Can you work these out from the model? Positions are in its coordinate system, mm. Round coordinates to 2 decimals unless told otherwise and drop trailing zeros. Loops run counter-clockwise (first coordinate to the right, second up) from the corner with the lowest first, then second, coordinate; pieces in that order, holes last. Notation, with made-up numbers: (16.5, -39.5) -> (75.5, -39.5) arc R28 ccw to (75.5, -15.5) -> close; hole circle Ø3 at (32.25, 39). An arc over 180 degrees is marked (long way). Write each question's results on one line, items separated by ' | '.
Autodesk Inventor part; units mm, degrees
ref_plane "YZ Plane" through (0, 0, 0) normal (1, 0, 0) x (0, 1, 0)
ref_plane "XZ Plane" through (0, 0, 0) normal (0, 1, 0) x (-1, 0, 0)
ref_plane "XY Plane" through (0, 0, 0) normal (0, 0, 1) x (1, 0, 0)
sketch "草圖1" plane through (0, 0, 0) normal (1, 0, 0) x (0, 1, 0)
  line L0 (-25, 50) -> (25, 50)
  line L1 (25, 50) -> (25, -50)
  line L2 (25, -50) -> (-25, -50)
  line L3 (-25, -50) -> (-25, 50)
  line L4 (-25, 50) -> (25, -50) construction
  line L5 (25, 50) -> (-25, -50) construction
  point P0 (0, 0)
  dimension "d0" = 50
  dimension "d1" = 100
extrude "擠出1" add sketch "草圖1" along normal blind 10
fillet "圓角1" radius 1 4 edges at (5, 25, 50) (5, -25, 50) (5, 25, -50) (5, -25, -50)
chamfer "倒角1" distance 1 angle 45 8 edges at (10, -25, 0) (10, -24.7071, -49.7071) (10, 0, -50) (10, 24.7071, -49.7071) (10, 25, 0) (10, 24.7071, 49.7071) (10, 0, 50) (10, -24.7071, 49.7071)
sketch "草圖2" plane through (10, 0, 0) normal (1, 0, 0) x (0, 0, -1)
  line L0 (-50, 24) -> (-50, -24)
  line L1 (49, 25) -> (-49, 25)
  line L2 (-30, 24) -> (-30, -24)
  line L3 (50, -24) -> (50, 24)
  line L4 (30, -24) -> (30, 24)
  line L5 (30, -12.5) -> (-30, -12.5)
  line L6 (-30, -12.5) -> (-30, 12.5)
  line L7 (-30, 12.5) -> (30, 12.5)
  line L8 (30, 12.5) -> (30, -12.5)
  line L9 (30, -12.5) -> (-30, 12.5) construction
  line L10 (-30, -12.5) -> (30, 12.5) construction
  point P0 (0, 0)
  dimension "d8" = 20
  dimension "d9" = 20
  dimension "d10" = 25
hole "孔1" at (10, 12.5, 30) at (10, -12.5, 30) at (10, 12.5, -30) at (10, -12.5, -30) direction (-1, 0, 0) diameter 10 end through all
thread "螺紋1"
thread "螺紋2"
chamfer "倒角2" distance 0.5 angle 45 8 edges at (10, -12.5, -25) (10, 12.5, -25) (10, -12.5, 35) (10, 12.5, 35) (0, -12.5, -25) (0, 12.5, -25) (0, -12.5, 35) (0, 12.5, 35)
properties part number "exercise3-3"
1. Please list where these lines run through material, in increasing order: line 1 (Y direction, x = 2.75, z = -30); line 2 (Z direction, x = 5.5, y = -12.5); line 3 (Z direction, x = 2.5, y = 10). Write a range as from..to.
Final values:
line 1: -25..-17.5, -7.5..7.5, 17.5..25 | line 2: -50..-35, -25..25, 35..50 | line 3: -50..-34.33, -25.67..25.67, 34.33..50
2. We'd pull the mould along Y, two halves only. Please class faces 1 (the face through (4, -25, -1)), 2 (the face through (4.937, -12.72, -25.005)), 3 (the face through (10, 0, 1)): pulls with the +Y half, pulls with the -Y half, needs draft (parallel to the pull), parting line crosses it, or undercut.
Final values:
face 1: pulls with the -Y half | face 2: undercut | face 3: needs draft
3. If we section it at A-A (z = -30): List the corners of the cut face in (x, y) for me, then the cut area to 3 significant figures.
Final values:
outline: (0, -25) -> (9, -25) -> (10, -24) -> (10, -18) -> (9.5, -17.5) -> (0.5, -17.5) -> (0, -18) -> close; (0, -7) -> (0.5, -7.5) -> (9.5, -7.5) -> (10, -7) -> (10, 7) -> (9.5, 7.5) -> (0.5, 7.5) -> (0, 7) -> close; (0, 18) -> (0.5, 17.5) -> (9.5, 17.5) -> (10, 18) -> (10, 24) -> (9, 25) -> (0, 25) -> close | area: 298 mm2
4. If we section it at C-C (x = 6.75): List the corners of the cut face in (y, z) for me, then the cut area to 3 significant figures.
Final values:
outline: (-25, -49) arc R1 ccw to (-24, -50) -> (24, -50) arc R1 ccw to (25, -49) -> (25, 49) arc R1 ccw to (24, 50) -> (-24, 50) arc R1 ccw to (-25, 49) -> close; hole circle Ø10 at (-12.5, -30); hole circle Ø10 at (-12.5, 30); hole circle Ø10 at (12.5, -30); hole circle Ø10 at (12.5, 30) | area: 4,680 mm2
5. Will this pin go through, and if not, where does the flat tip stop? pin 1 (2 mm diameter, centred on y = -8.5, z = -29.5, fed in from +X).
Final values:
pin 1: x = 9.53
6. If we section it at B-B (y = -12.5): List the corners of the cut face in (x, z) for me.
Final values:
outline: (0, -50) -> (9, -50) -> (10, -49) -> (10, -35.5) -> (9.5, -35) -> (0.5, -35) -> (0, -35.5) -> close; (0, -24.5) -> (0.5, -25) -> (9.5, -25) -> (10, -24.5) -> (10, 24.5) -> (9.5, 25) -> (0.5, 25) -> (0, 24.5) -> close; (0, 35.5) -> (0.5, 35) -> (9.5, 35) -> (10, 35.5) -> (10, 49) -> (9, 50) -> (0, 50) -> close
